CAD build for the part. Positions are in the model's coordinates, mm. A direction names the side the tool comes from. Round coordinates to 2 decimals unless told otherwise and drop trailing zeros. Loops run counter-clockwise (first coordinate to the right, second up) from the corner with the lowest first, then second, coordinate; pieces in that order, holes last. Notation, with made-up numbers: M 12.25,78.5 L 35.25,78.5 A22 ccw 35.25,92.5 Z; hole C 38,-25 d2. An arc over 180 degrees is marked long. Use a Markdown table: item, result. Add a question column.
(1) Band-saw the part on A-A, the plane y = -13. Give the number of separate pieces and of enclosed holes in the cut face, and give its area (3 significant figures).
(2) Wall check: L1, parallel to X at y = 23, z = -15.5; L2, parallel to Y at x = -23, z = -10; L3, parallel to X at y = 18, z = -15.5. Give the ranges that are in metal, low to high.
(3) Band-saw the part on D-D, the plane y = 9. Write the cut outline in (x, z), and give its area (3 significant figures).
(4) Flat gauge pins, fed straight in: P1, Ø12, axis at x = -1.5, z = 19.5, coming from the +Y side; P2, Ø9.5, axis at x = -23, y = 23, coming from the -Z side; P3, Ø3, axis at y = -23, z = 31, coming from the +X side. Where does each tip first touch, or does it go through?
(5) Band-saw the part on C-C, the plane x = 23. Write the cut outline in (y, z).
(6) Which spindle directions (+Z, -Z, +X, -X, +Y, -Y) get a long thin tool onto all of the face, cutting with end or side? Do faces 5 (the face through (-8.296, -2.81, 34.488)), 6 (the face through (-39, -6, 12)), 7 (the face through (-4, 15, 16)). Say none if no direction does.
(7) Band-saw the part on B-B, the plane z = -2. Write the cut outline in (x, y), and give its area (3 significant figures).
(8) Two-plate mould, pull along Z, no slides. Class faces 1 (the face through (13, -29, 51)), 2 (the face through (-41, -29, 6)), 3 (the face through (-6.474, -4.266, 12.401)), 4 (the face through (0, 35, -10)): released by +Z, released by -Z, zero draft, split by the parting line, or undercut.
from build123d import *

# Parameters (mm, degrees)
BOSS_EXTRUDE1_DEPTH       = 35
BOSS_EXTRUDE2_DEPTH       = 12
BOSS_EXTRUDE3_DEPTH       = 12
SKETCH4_R                 = 19
BOSS_EXTRUDE4_DEPTH       = 20
BOSS_EXTRUDE5_DEPTH       = 38
SKETCH7_W                 = 6
SKETCH7_H                 = 100
LPATTERN1_COUNT           = 2
LPATTERN1_PITCH           = 33
LPATTERN2_COUNT           = 2
LPATTERN2_PITCH           = 46
LPATTERN2_COPY_1_SKETCH_W = 6
LPATTERN2_COPY_1_SKETCH_H = 100
SKETCH8_R                 = 3
CUT_EXTRUDE1_DEPTH        = 108.736551619


with BuildPart() as part:
    # Sketch1 → Boss-Extrude1 (new, symmetric)
    with BuildSketch(Plane(origin=(0, 0, 0), x_dir=(1, 0, 0), z_dir=(0, 1, 0))):
        Polygon((-10, 20), (-10, 17), (10, 17), (10, 20), (35, 20), (35, 0), (-35, 0), (-35, 20), align=None)
    extrude(amount=BOSS_EXTRUDE1_DEPTH, both=True)

    # Sketch2 → Boss-Extrude2 (add)
    with BuildSketch(Plane(origin=(0, -35, 0), x_dir=(-1, 0, 0), z_dir=(0, -1, 0))):
        with BuildLine():
            Line((-35, 0), (35, 0))
            Line((35, 0), (47.377416998, -12.377416998))
            Line((47.377416998, -12.377416998), (-2.121320344, -61.876154339))
            Line((-2.121320344, -61.876154339), (-24.748737342, -39.248737342))
            ThreePointArc((-24.748737342, -39.248737342), (-32.335783638, -27.893920133), (-35, -14.5))
            Line((-35, -14.5), (-35, 0))
        make_face()
    extrude(amount=-BOSS_EXTRUDE2_DEPTH)

    # Sketch3 → Boss-Extrude3 (add)
    with BuildSketch(Plane(origin=(-29.877416998, 0, 29.877416998), x_dir=(0.7071067811865468, 0, 0.7071067811865482), z_dir=(-0.7071067811865482, 0, 0.7071067811865468))):
        with BuildLine():
            Line((-24.748737342, -23), (-13.468721173, 10.894302389))
            ThreePointArc((-13.468721173, 10.894302389), (10.252155493, 28), (33.973032159, 10.894302389))
            Line((33.973032159, 10.894302389), (45.253048327, -23))
            Line((45.253048327, -23), (-24.748737342, -23))
        make_face()
    extrude(amount=-BOSS_EXTRUDE3_DEPTH)

    # Sketch4 → Boss-Extrude4 (add)
    with BuildSketch(Plane(origin=(-29.877416998, 0, 29.877416998), x_dir=(0.7071067811865468, 0, 0.7071067811865482), z_dir=(-0.7071067811865482, 0, 0.7071067811865468))):
        with Locations((10.252155493, 3)):
            Circle(SKETCH4_R)
    extrude(amount=BOSS_EXTRUDE4_DEPTH)

    # Sketch5 → Boss-Extrude5 (add)
    with BuildSketch(Plane(origin=(0, -23, 0), x_dir=(1, 0, 0), z_dir=(0, 1, 0))):
        with BuildLine():
            Line((-6, 0), (-6, -10.063607341))
            ThreePointArc((-6, -10.063607341), (-6.487174562, -12.431888509), (-7.869585231, -14.415580897))
            Line((-7.869585231, -14.415580897), (-18.386854658, -24.39741659))
            Line((-18.386854658, -24.39741659), (-9.898679248, -32.885591999))
            Line((-9.898679248, -32.885591999), (0.391244308, -23.119528009))
            ThreePointArc((0.391244308, -23.119528009), (4.538476314, -17.168450846), (6, -10.063607341))
            Line((6, -10.063607341), (6, 0))
            Line((6, 0), (-6, 0))
        make_face()
    extrude(amount=BOSS_EXTRUDE5_DEPTH)

    # Sketch7 → Hole1 (revolve, cut)
    with BuildSketch(Plane(origin=(23, -10, 0), x_dir=(0, -1, 0), z_dir=(1, 0, 0))):
        with Locations((3, 50)):
            Rectangle(SKETCH7_W, SKETCH7_H)
    hole1 = revolve(axis=Axis((23, -10, -110), (0, 0, 1)), mode=Mode.SUBTRACT)

    # LPattern1: Hole1 ×2
    with Locations(*[(0, i * LPATTERN1_PITCH, 0) for i in range(1, LPATTERN1_COUNT)]):
        add(hole1, mode=Mode.SUBTRACT)

    # LPattern2: Hole1 ×2
    with Locations(*[(-i * LPATTERN2_PITCH, 0, 0) for i in range(1, LPATTERN2_COUNT)]):
        add(hole1, mode=Mode.SUBTRACT)

    # LPattern2 copy 1 sketch → LPattern2 copy 1 (revolve, cut)
    with BuildSketch(Plane(origin=(-23, 23, 0), x_dir=(0, -1, 0), z_dir=(1, 0, 0))):
        with Locations((3, 50)):
            Rectangle(LPATTERN2_COPY_1_SKETCH_W, LPATTERN2_COPY_1_SKETCH_H)
    revolve(axis=Axis((-23, 23, -110), (0, 0, 1)), mode=Mode.SUBTRACT)

    # Sketch8 → Cut-Extrude1 (cut, through all)
    with BuildSketch(Plane(origin=(0, 35, 0), x_dir=(1, 0, 0), z_dir=(0, 1, 0))):
        with Locations(Location((-29.699116139, -44.197853481, 0), (0, 0, 270))):
            Circle(SKETCH8_R)
    extrude(amount=-CUT_EXTRUDE1_DEPTH, mode=Mode.SUBTRACT)


solid = part.part
Return value:
| question | item | result |
|---|---|---|
| 1 | separate pieces | 3 |
| 1 | enclosed holes | 1 |
| 1 | area | 2,480 mm^2 |
| 2 | L1 | -35 to -29, -17 to 17, 29 to 35 |
| 2 | L2 | -35 to -16, -4 to 17, 29 to 35 |
| 2 | L3 | -35 to -26.32, -19.68 to 19.68, 26.32 to 35 |
| 3 | outline | M -49.52,38.52 L -35.38,24.38 L -39.85,19.91 L -31.36,11.42 L -18.39,24.4 L -7.87,14.42 A6 cw -6,10.06 L -6,0 L -35,0 L -35,-20 L -10,-20 L -10,-17 L 10,-17 L 10,-20 L 35,-20 L 35,0 L 6,0 L 6,10.06 A18 ccw 0.39,23.12 L -9.9,32.89 L 3.08,45.86 L -5.41,54.35 L -9.88,49.87 L -24.02,64.02 Z; hole C -29.7,44.2 d6 |
| 3 | area | 3,030 mm^2 |
| 4 | P1 | y = 15 |
| 4 | P2 | z = 15.88 |
| 4 | P3 | x = 31.62 |
| 5 | outline | M -35,-20 L -16,-20 L -16,0 L -23,0 L -23,41 L -35,41 Z; M -4,-20 L 17,-20 L 17,0 L -4,0 Z; M 29,-20 L 35,-20 L 35,0 L 29,0 Z |
| 6 | face 5 | +Y |
| 6 | face 6 | -X, +Y |
| 6 | face 7 | +X, +Y |
| 7 | outline | M -35,-35 L 35,-35 L 35,35 L -35,35 Z; hole C -23,-10 d12; hole C -23,23 d12; hole C 23,-10 d12; hole C 23,23 d12 |
| 7 | area | 4,450 mm^2 |
| 8 | face 1 | released by +Z |
| 8 | face 2 | released by -Z |
| 8 | face 3 | undercut |
| 8 | face 4 | zero draft |
